The listing builds one solid part. Answer for the finished solid, in the listing's coordinates (mm). A direction names the side the tool comes from. Round coordinates to 2 decimals unless told otherwise and drop trailing zeros. Write each loop counter-clockwise with the first axis right and the second up, starting at its lowest first coordinate (ties: lowest second). Pieces come first, ordered by that corner, then holes.
Item 1: This flat-tipped pin is pushed along its axis until it touches: pin 1 (3 mm diameter, centred on x = -15.5, y = 7, fed in from +Z). Where does it stop, or does it pass through?
Item 2: Find section A-A on z = 84.5. Give the vertices of the cut face in (x, y).
Item 3: Find section D-D on z = 103.5. Give the vertices of the cut face in (x, y).
Item 4: Find section C-C on y = 15.5. Give the vertices of the cut face in (x, z), then the cut area to 3 significant figures.
Item 5: Find section B-B on x = 7.5. Give the vertices of the cut face in (y, z).
Item 6: A tool of negligible diameter and unlimited length cuts with its end or side. For faces 1 (the face through (7.11, 36.58, 1.5)), 2 (the face through (13.55, -7, 107.4)), 3 (the face through (-25.719, -42.587, 49.905)), from which of +Z, -Z, +X, -X, +Y, -Y can it reach the whole face along a straight path? Write none if from no direction.
Item 7: For a pull along Z with two mould halves and no side action, classify faces 4 (the face through (7.115, 36.504, 98.574)), 5 (the face through (8, 36.007, 50)), 6 (the face through (-29, -5, 2)) as +Z half, -Z half, draft (parallel to the pull), parting line (faces both ways), or undercut.
Item 8: Find the intervals of material crossed by probe 1 along Z at (x, y) = (-16.5, -4); probe 2 along X at (y, z) = (-36, 26.5); probe 3 along Y at (x, z) = (18.5, 62), in increasing order.
```python
from build123d import *

# Parameters (mm, degrees)
BOSS_EXTRUDE1_DEPTH = 100
BOSS_EXTRUDE2_DEPTH = 3
BOSS_EXTRUDE3_START = -2
BOSS_EXTRUDE3_DEPTH = 2
FILLET2_R           = 5
SKETCH5_R           = 9.55
SKETCH5_R_2         = 6.55
BOSS_EXTRUDE4_DEPTH = 15


with BuildPart() as part:
    # Sketch1 → Boss-Extrude1 (new body)
    with BuildSketch(Plane.XY):
        with BuildLine():
            Line((-20, -46.992716482), (35, -46.992716482))
            ThreePointArc((35, -46.992716482), (42.071067812, -44.063784293), (45, -36.992716482))
            Line((45, -36.992716482), (45, 28.007283518))
            ThreePointArc((45, 28.007283518), (42.071067812, 35.07835133), (35, 38.007283518))
            Line((35, 38.007283518), (-20, 38.007283518))
            ThreePointArc((-20, 38.007283518), (-27.071067812, 35.07835133), (-30, 28.007283518))
            Line((-30, 28.007283518), (-30, -36.992716482))
            ThreePointArc((-30, -36.992716482), (-27.071067812, -44.063784293), (-20, -46.992716482))
        make_face()
        with BuildLine():
            Line((-20, -44.992716482), (35, -44.992716482))
            ThreePointArc((35, -44.992716482), (40.656854249, -42.649570731), (43, -36.992716482))
            Line((43, -36.992716482), (43, 28.007283518))
            ThreePointArc((43, 28.007283518), (40.656854249, 33.664137768), (35, 36.007283518))
            Line((35, 36.007283518), (-20, 36.007283518))
            ThreePointArc((-20, 36.007283518), (-25.656854249, 33.664137768), (-28, 28.007283518))
            Line((-28, 28.007283518), (-28, -36.992716482))
            ThreePointArc((-28, -36.992716482), (-25.656854249, -42.649570731), (-20, -44.992716482))
        make_face(mode=Mode.SUBTRACT)
    extrude(amount=BOSS_EXTRUDE1_DEPTH)

    # Sketch2 → Boss-Extrude2 (add)
    with BuildSketch(Plane(origin=(0, 0, 0), x_dir=(-1, 0, 0), z_dir=(0, 0, -1))):
        with BuildLine():
            Line((-35, -46.992716482), (20, -46.992716482))
            ThreePointArc((20, -46.992716482), (27.071067812, -44.063784293), (30, -36.992716482))
            Line((30, -36.992716482), (30, 28.007283518))
            ThreePointArc((30, 28.007283518), (27.071067812, 35.07835133), (20, 38.007283518))
            Line((20, 38.007283518), (-35, 38.007283518))
            ThreePointArc((-35, 38.007283518), (-42.071067812, 35.07835133), (-45, 28.007283518))
            Line((-45, 28.007283518), (-45, -36.992716482))
            ThreePointArc((-45, -36.992716482), (-42.071067812, -44.063784293), (-35, -46.992716482))
        make_face()
    extrude(amount=-BOSS_EXTRUDE2_DEPTH)

    # Sketch4 → Boss-Extrude3 (add)
    with BuildSketch(Plane.XY.offset(100).offset(BOSS_EXTRUDE3_START)):
        with BuildLine():
            Line((-20, -46.992716482), (35, -46.992716482))
            ThreePointArc((35, -46.992716482), (42.071067812, -44.063784293), (45, -36.992716482))
            Line((45, -36.992716482), (45, 28.007283518))
            ThreePointArc((45, 28.007283518), (42.071067812, 35.07835133), (35, 38.007283518))
            Line((35, 38.007283518), (-20, 38.007283518))
            ThreePointArc((-20, 38.007283518), (-27.071067812, 35.07835133), (-30, 28.007283518))
            Line((-30, 28.007283518), (-30, -36.992716482))
            ThreePointArc((-30, -36.992716482), (-27.071067812, -44.063784293), (-20, -46.992716482))
        make_face()
    extrude(amount=BOSS_EXTRUDE3_DEPTH)

    # Fillet2
    fillet2_edges = [part.edges().sort_by_distance(p)[0] for p in [
        (7.5, 38.007283518, 0),
        (-28, -4.492716482, 98),
        (-25.656854249, -42.649570731, 98),
        (7.5, -44.992716482, 98),
        (40.656854249, -42.649570731, 98),
        (43, -4.492716482, 98),
        (40.656854249, 33.664137768, 98),
        (42.071067812, 35.07835133, 0),
        (7.5, 36.007283518, 98),
        (-25.656854249, 33.664137768, 98),
        (45, -4.492716482, 0),
        (42.071067812, -44.063784293, 0),
        (42.071067812, 35.07835133, 100),
        (7.5, 38.007283518, 100),
        (-27.071067812, 35.07835133, 100),
        (-30, -4.492716482, 100),
        (-27.071067812, -44.063784293, 100),
        (7.5, -46.992716482, 100),
        (42.071067812, -44.063784293, 100),
        (-28, -4.492716482, 3),
        (7.5, -44.992716482, 3),
        (-25.656854249, -42.649570731, 3),
        (-25.656854249, 33.664137768, 3),
        (7.5, 36.007283518, 3),
        (40.656854249, 33.664137768, 3),
        (43, -4.492716482, 3),
        (40.656854249, -42.649570731, 3),
        (7.5, -46.992716482, 0),
        (45, -4.492716482, 100),
        (-27.071067812, -44.063784293, 0),
        (-30, -4.492716482, 0),
        (-27.071067812, 35.07835133, 0),
    ]]
    fillet(fillet2_edges, radius=FILLET2_R)

    # Sketch5 → Boss-Extrude4 (add)
    with BuildSketch(Plane.XY.offset(100)):
        with Locations((7.5, -4.492716482)):
            Circle(SKETCH5_R)
        with Locations((7.5, -4.492716482)):
            Circle(SKETCH5_R_2, mode=Mode.SUBTRACT)
    extrude(amount=BOSS_EXTRUDE4_DEPTH)


solid = part.part
```
Check values:
1. pin 1: stops at z = 100
2. outline: (-30, -36.99) arc R10 ccw to (-20, -46.99) - (35, -46.99) arc R10 ccw to (45, -36.99) - (45, 28.01) arc R10 ccw to (35, 38.01) - (-20, 38.01) arc R10 ccw to (-30, 28.01) - close; hole (-28, -36.99) arc R8 ccw to (-20, -44.99) - (35, -44.99) arc R8 ccw to (43, -36.99) - (43, 28.01) arc R8 ccw to (35, 36.01) - (-20, 36.01) arc R8 ccw to (-28, 28.01) - close
3. outline: circle Ø19.1 at (7.5, -4.49); hole circle Ø13.1 at (7.5, -4.49)
4. outline: (-30, 5) arc R5 ccw to (-25, 0) - (40, 0) arc R5 ccw to (45, 5) - (45, 95) arc R5 ccw to (40, 100) - (-25, 100) arc R5 ccw to (-30, 95) - close; hole (-28, 8) arc R5 ccw to (-23, 3) - (38, 3) arc R5 ccw to (43, 8) - (43, 93) arc R5 ccw to (38, 98) - (-23, 98) arc R5 ccw to (-28, 93) - close
4. area: 755 mm2
5. outline: (-46.99, 5) arc R5 ccw to (-41.99, 0) - (33.01, 0) arc R5 ccw to (38.01, 5) - (38.01, 95) arc R5 ccw to (33.01, 100) - (5.06, 100) - (5.06, 115) - (2.06, 115) - (2.06, 100) - (-11.04, 100) - (-11.04, 115) - (-14.04, 115) - (-14.04, 100) - (-41.99, 100) arc R5 ccw to (-46.99, 95) - close; hole (-44.99, 8) arc R5 ccw to (-39.99, 3) - (31.01, 3) arc R5 ccw to (36.01, 8) - (36.01, 93) arc R5 ccw to (31.01, 98) - (-39.99, 98) arc R5 ccw to (-44.99, 93) - close
6. face 1: -Z, +X, -X, +Y
6. face 2: +Z
6. face 3: none
7. face 4: +Z half
7. face 5: undercut
7. face 6: -Z half
8. probe 1: z = 0 to 3, 98 to 100
8. probe 2: x = -30 to -28, 43 to 45
8. probe 3: y = -46.99 to -44.99, 36.01 to 38.01
